Geometry check sheet. Reference: the model listing, model coordinates, mm. Face numbers are marked on the shaded views. A direction names the side the tool comes from. Give positions to 0.01 mm unless a question says otherwise; leave off trailing zeros. Write each loop counter-clockwise with the first axis right and the second up, starting at its lowest first coordinate (ties: lowest second). Pieces come first, ordered by that corner, then holes. Notation, with made-up numbers: (42.5, 43) - (63.5, 43) arc R19 cw to (63.5, 69) - close; hole circle Ø10 at (66, 61.25). An arc over 180 degrees is marked (long way). Write item = value, one per line. Start each with the question number.
(1) Depth check by flat-ended pin: pin 1 Ø4.5 at (y, z) = (46.02, 62.71) entering from -X; pin 2 Ø6 at (y, z) = (4.78, 62.71) entering from +X. Enter the tip coordinate at first touch or a pass-through.
(2) Access from +Z, -Z, +X, -X, +Y, -Y to the whole of each face (thin tool, end or side, straight path). Record for the marked faces 1 and 2.
(3) Section check A-A, the plane z = 50.8. Enter the section's corners in (x, y) (3 decimals).
(4) Section check B-B, the plane z = 299. Enter the section's corners in (x, y).
(5) Thickness scan on L1, parallel to Z at x = -25.4, y = 0.3; L2, parallel to X at y = 27, z = 320.5; L3, parallel to Y at x = -9.5, z = 351.5. Record the ranges inside material, lowest first.
Autodesk Inventor part; units mm, degrees
ref_plane "YZ Plane" through (0, 0, 0) normal (1, 0, 0) x (0, 1, 0)
ref_plane "XZ Plane" through (0, 0, 0) normal (0, 1, 0) x (-1, 0, 0)
ref_plane "XY Plane" through (0, 0, 0) normal (0, 0, 1) x (1, 0, 0)
sketch "Sketch1" plane through (0, 0, 0) normal (0, 0, 1) x (1, 0, 0)
  line L0 (0, 0) -> (-50.8, 0)
  line L1 (-50.8, 0) -> (-50.8, 50.8)
  line L2 (-50.8, 50.8) -> (0, 50.8)
  line L3 (0, 50.8) -> (0, 0)
  line L4 (-49.149, 49.149) -> (-1.651, 49.149)
  line L5 (-1.651, 49.149) -> (-1.651, 1.651)
  line L6 (-1.651, 1.651) -> (-49.149, 1.651)
  line L7 (-49.149, 1.651) -> (-49.149, 49.149)
  dimension "d0" = 50.8
  dimension "d1" = 50.8
  dimension "d2" = 1.651
  dimension "d3" = 1.651
  dimension "d4" = 1.651
  dimension "d5" = 1.651
extrude "Extrusion1" add sketch "Sketch1" along normal blind 431.8
sketch "Sketch2" plane through (-50.8, 0, 0) normal (-1, 0, 0) x (0, 0, 1)
  circle A0 centre (114.3, 38.1) radius 2.5797
  circle A1 centre (139.7, 38.1) radius 2.5797
  circle A2 centre (165.1, 38.1) radius 2.5797
  circle A3 centre (368.3, 38.1) radius 2.5797
  circle A4 centre (393.7, 38.1) radius 2.5797
  circle A5 centre (419.1, 38.1) radius 2.5797
  line L0 (0, 0) -> (0, 50.8)
  line L1 (431.8, 50.8) -> (431.8, 0)
  line L2 (0, 50.8) -> (431.8, 50.8)
  dimension "d8" = 114.3
  dimension "d9" = 25.4
  dimension "d10" = 25.4
  dimension "d11" = 25.4
  dimension "d12" = 25.4
  dimension "d13" = 12.7
  dimension "d14" = 5.1594
  dimension "d15" = 5.1594
  dimension "d16" = 5.1594
  dimension "d19" = 5.1594
  dimension "d20" = 5.1594
  dimension "d21" = 5.1594
  dimension "d22" = 12.7
  dimension "d23" = 12.7
  dimension "d24" = 12.7
  dimension "d25" = 12.7
  dimension "d26" = 12.7
  dimension "d27" = 12.7
extrude "Extrusion2" cut sketch "Sketch2" against normal blind 279.4
sketch "Sketch5" plane through (0, 0, 0) normal (1, 0, 0) x (0, 0, -1)
  circle A0 centre (-50.8, 25.4) radius 9.525
  circle A1 centre (-26.9875, 25.4) radius 2.5797
  line L0 (0, 50.8) -> (0, 0)
  circle A2 centre (-50.8, 25.4) radius 23.8125 construction
  line L1 (0, 0) -> (-431.8, 0)
  circle A3 centre (-50.8, 25.4) radius 23.8125 construction
  circle A4 centre (-38.8938, 46.0222) radius 2.5797
  circle A5 centre (-50.8, 25.4) radius 23.8125 construction
  circle A6 centre (-62.7062, 46.0222) radius 2.5797
  circle A7 centre (-50.8, 25.4) radius 23.8125 construction
  circle A8 centre (-74.6125, 25.4) radius 2.5797
  circle A9 centre (-50.8, 25.4) radius 23.8125 construction
  circle A10 centre (-62.7063, 4.7778) radius 2.5797
  circle A11 centre (-50.8, 25.4) radius 23.8125 construction
  circle A12 centre (-38.8938, 4.7778) radius 2.5797
  dimension "d36" = 50.8
  dimension "d37" = 23.8125
  dimension "d38" = 19.05
  dimension "d39" = 5.1594
  dimension "d40" = 25.4
  dimension "d41" = 25.4
  dimension "d44" = 360
extrude "Extrusion4" cut sketch "Sketch5" against normal blind 50.8 contours A1 | A4 | A6 | A8 | A10 | A12
sketch "Sketch6" plane through (0, 0, 0) normal (1, 0, 0) x (0, 0, -1)
  circle A0 centre (-50.8, 25.4) radius 14.605
  line L0 (0, 0) -> (-431.8, 0)
  circle A1 centre (-26.9875, 25.4) radius 2.5797
  dimension "d48" = 25.4
  dimension "d49" = 23.8125
  dimension "d50" = 29.21
extrude "Extrusion5" cut sketch "Sketch6" against normal blind 50.8 contours A0
sketch "Sketch7" plane through (-50.8, 0, 0) normal (0, -1, 0) x (1, 0, 0)
  circle A0 centre (12.7, 419.1) radius 2.5797
  circle A1 centre (38.1, 419.1) radius 2.5797
  line L0 (49.149, 0) -> (49.149, 431.8)
  line L1 (0, 431.8) -> (50.8, 431.8)
  circle A2 centre (25.4, 419.1) radius 2.5797
  line L2 (50.8, 0) -> (50.8, 431.8)
  line L3 (38.1, 419.1) -> (38.1, 368.3) construction
  line L4 (38.1, 419.1) -> (88.9, 419.1) construction
  line L5 (25.4, 419.1) -> (25.4, 368.3) construction
  line L6 (12.7, 419.1) -> (12.7, 368.3) construction
  circle A3 centre (38.1, 368.3) radius 2.5797
  circle A4 centre (25.4, 368.3) radius 2.5797
  circle A5 centre (12.7, 368.3) radius 2.5797
  dimension "d53" = 5.1594
  dimension "d54" = 25.4
  dimension "d56" = 12.7
  dimension "d57" = 5.1594
  dimension "d58" = 5.1594
  dimension "d59" = 12.7
  dimension "d60" = 25.4
  dimension "d61" = 12.7
  dimension "d62" = 12.7
  dimension "d65" = 50.8
  dimension "d66" = 90
  dimension "d67" = 50.8
  dimension "d68" = 50.8
  dimension "d69" = 5.1594
  dimension "d70" = 5.1594
  dimension "d71" = 5.1594
extrude "Extrusion7" cut sketch "Sketch7" against normal blind 127
equation "\"d3\" = d2"
equation "\"d4\" = d2"
equation "\"d5\" = d2"
equation "\"d10\" = d9"
equation "\"d11\" = d9"
equation "\"d15\" = d14"
equation "\"d16\" = d14"
equation "\"d19\" = d14"
equation "\"d20\" = d14"
equation "\"d21\" = d14"
equation "\"d26\" = d25"
equation "\"d27\" = d25"
equation "\"d57\" = d53"
equation "\"d58\" = d57"
properties part number "ATACHMENT BAR"
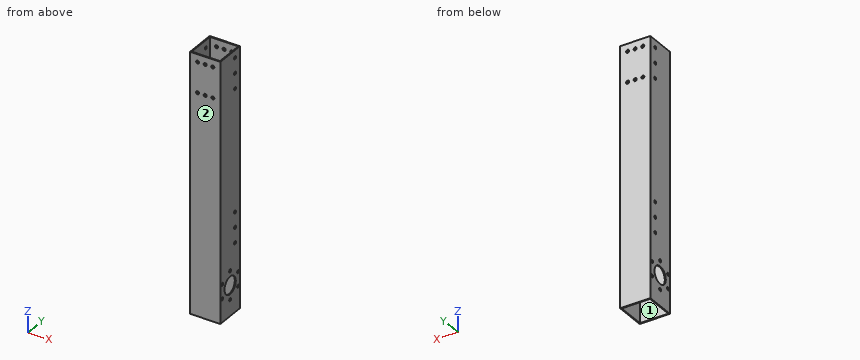
Model answer:
q1.pin_1 = through
q1.pin_2 = 0
q2.face_1 = +Z, -Z
q2.face_2 = +Z, -Z, +X, -X, -Y
q3.outline = (-50.8, 0) - (0, 0) - (0, 10.795) - (-1.651, 10.795) - (-1.651, 1.651) - (-49.149, 1.651) - (-49.149, 10.795) - (-50.8, 10.795) - close; (-50.8, 40.005) - (-49.149, 40.005) - (-49.149, 49.149) - (-1.651, 49.149) - (-1.651, 40.005) - (0, 40.005) - (0, 50.8) - (-50.8, 50.8) - close
q4.outline = (-50.8, 0) - (0, 0) - (0, 50.8) - (-50.8, 50.8) - close; hole (-49.15, 1.65) - (-1.65, 1.65) - (-1.65, 49.15) - (-49.15, 49.15) - close
q5.L1 = 0 to 365.72, 370.88 to 416.52, 421.68 to 431.8
q5.L2 = -50.8 to -49.15, -1.65 to 0
q5.L3 = 0 to 1.65, 49.15 to 50.8
